Autodesk Fusion 360 part; units mm, degrees
sketch "Sketch1" plane through (0, 0, 0) normal (0, 0, 1) x (1, 0, 0)
  circle A0 centre (0, 0) radius 6
  circle A1 centre (0, 0) radius 1
  dimension "d1" = 2
  dimension "d12" = 12
extrude "Extrude1" add sketch "Sketch1" along normal blind 10
sketch "Sketch2" plane through (0, 0, 0) normal (1, 0, 0) x (0, 1, 0)
  circle A0 centre (0, 4.686) radius 1.55
  dimension "d4" = 3.1
extrude "Extrude2" cut sketch "Sketch2" along normal blind 12
sketch "Sketch3" plane through (0, 0, 10) normal (0, 0, 1) x (-1, 0, 0)
  circle A0 centre (0, 0) radius 1
  circle A1 centre (0, 0) radius 6
  line L0 (-2, 0.003) -> (-2, 3.003)
  line L1 (-2, 0.003) -> (-2, -2.997)
  line L2 (-2, 3.003) -> (-4.5, 3.003)
  line L3 (-2, -2.997) -> (-4.5, -2.997)
  line L4 (-4.5, 3.003) -> (-4.5, -2.997)
  dimension "d7" = 3
  dimension "d8" = 3
  dimension "d9" = 2.5
  dimension "d10" = 2.5
  dimension "d11" = 2
extrude "Extrude3" [suppressed]
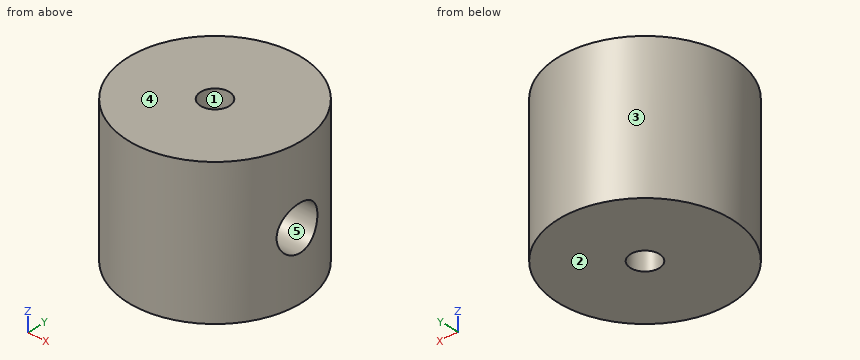
The model under review builds one solid part; all positions refer to its coordinate system, in mm. Face numbers are marked on the shaded views. A direction names the side the tool comes from. Give positions to 0.01 mm unless a question says otherwise; leave off trailing zeros. Write each loop counter-clockwise with the first axis right and the second up, starting at its lowest first coordinate (ties: lowest second). Pieces come first, ordered by that corner, then holes. Notation, with made-up numbers: M -15,52 L 29,52 A21 cw 29,71 Z; hole C -36.75,30 d3. An arc over 180 degrees is marked long. Write item = value, one per line. Start each with the question number.
Q1. We need section B-B (x = 2.25). State the section outline as (y, z) points, plus the area to 3 significant figures.
Q2. Mouldability with a two-part tool opening along X and no side actions: class the marked faces 1, 2 and 3 as released by +X, released by -X, zero draft, split by the parting line, or undercut.
Q3. Clearance check with flat-ended pins moving along their axes: pin 1 (3 mm diameter, centred on x = 3, z = 6.5, fed in from -Y); pin 2 (6 mm diameter, centred on y = 3.5, z = 8.5, fed in from -X); pin 3 (0.6 mm diameter, centred on y = -1.5, z = 5, fed in from +X). State where each tip first meets the part, or that it passes through.
Q4. Machinability: for the marked faces 4 and 5, which of the approach directions +Z, -Z, +X, -X, +Y, -Y give a long, thin tool a straight path to every point of the face, cutting with its end or side? Answer none if there is none.
Q5. We need section D-D (z = 5.5). State the section outline as (x, y) points, plus the area to 3 significant figures.
Q6. We need section A-A (y = 0.5). State the section outline as (x, z) points, plus the area to 3 significant figures.
Q7. We need section C-C (z = 0.5). State the section outline as (x, y) points, plus the area to 3 significant figures.
Q8. For line 1 (Z direction, x = 2.25, y = 0); line 2 (Z direction, x = 4.25, y = -1); line 3 (Y direction, x = 1, z = 4.75), list the stretches that pass through material, from the lowest coordinate up.
Result set:
q1.outline = M -5.56,0 L 5.56,0 L 5.56,10 L -5.56,10 Z; hole C 0,4.69 d3.1
q1.area = 104 mm2
q2.face_1 = undercut
q2.face_2 = zero draft
q2.face_3 = split by the parting line
q3.pin_1 = -5.81
q3.pin_2 = -5.98
q3.pin_3 = 5.83
q4.face_4 = +Z, +X, -X, +Y, -Y
q4.face_5 = +X
q5.outline = M 0,-1.32 L 0,-1 A1 cw 0,1 L 0,1.32 L 5.85,1.32 A6 ccw long 5.85,-1.32 Z
q5.area = 95.8 mm2
q6.outline = M -5.98,0 L -0.87,0 L -0.87,10 L -5.98,10 Z; M 0.87,0 L 5.98,0 L 5.98,3.22 L 0.87,3.22 Z; M 0.87,6.15 L 5.98,6.15 L 5.98,10 L 0.87,10 Z
q6.area = 87.3 mm2
q7.outline = C 0,0 d12; hole C 0,0 d2
q7.area = 110 mm2
q8.line_1 = 0 to 3.14, 6.24 to 10
q8.line_2 = 0 to 3.5, 5.87 to 10
q8.line_3 = -5.92 to -1.55, 1.55 to 5.92
